Input: part model. Units: mm. Frame: model coordinates. A direction names the side the tool comes from. Coordinates: 2 decimals unless noted, no trailing zeros. Loops run counter-clockwise (first coordinate to the right, second up) from the corner with the lowest first, then second, coordinate; pieces in that order, holes last.
Item 1: Section A-A on x = 32. Return loops of the section in (y, z), and give its area (3 significant figures).
Item 2: Reachability of faces 5 (the cylindrical face through (11.155, 12.58, 2.696)), 6 (the flat face through (38, 8, 3)), 7 (the flat face through (30, 8, 6.35)) from +Z, -Z, +X, -X, +Y, -Y: full face, straight path, thin tool, end or side. Return the list, or none.
Item 3: Section B-B on y = 7.5. Return loops of the section in (x, z).
Item 4: Section D-D on y = 13. Return loops of the section in (x, z) (3 decimals), and give its area (3 significant figures).
Item 5: Ray query, line 1 along Y through (x, z) = (40, 6); line 2 along X through (y, z) = (5.5, 1.5); line 3 along Z through (x, y) = (10, 13.4) (3 decimals). Return the intervals inside material, ascending.
Item 6: Contact query for a flat-ended pin moving along its axis: P1, Ø3, axis at x = 32, y = 2, coming from the +Z side. Output: stop coordinate, or through.
Item 7: Pull-direction query (Y, two-part tool) for faces 1 (the cylindrical face through (51.192, 12.58, 3.55)), 2 (the flat face through (30, 0, 3)), 3 (the flat face through (30, 15, 3)), 4 (the flat face through (39, 3.769, 3)); classes: released by +Y, released by -Y, zero draft, split by the parting line, or undercut.
Item 8: Section C-C on x = 40.5. Return loops of the section in (y, z), and give its area (4 significant figures).
```python
from build123d import *

# Parameters (mm, degrees)
SKETCH1_W             = 60
SKETCH1_H             = 15
SKETCH1_R             = 3
BOSS_EXTRUDE1_DEPTH   = 6.35
M3_TAPPED_HOLE1_D     = 2.5
M3_TAPPED_HOLE1_DEPTH = 8.5
M3_TAPPED_HOLE1_TIP   = 0.751075774
SKETCH5_W             = 3
SKETCH5_H             = 8
CUT_EXTRUDE1_DEPTH    = 63.171717881
M3_TAPPED_HOLE2_D     = 2.5


with BuildPart() as part:
    # Sketch1 → Boss-Extrude1 (new body)
    with BuildSketch(Plane.XY):
        with Locations((30, 7.5)):
            Rectangle(SKETCH1_W, SKETCH1_H)
        with Locations((10, 7.5)):
            Circle(SKETCH1_R, mode=Mode.SUBTRACT)
        with Locations(Location((50, 7.5, 0), (0, 0, 180))):
            Circle(SKETCH1_R, mode=Mode.SUBTRACT)
    extrude(amount=BOSS_EXTRUDE1_DEPTH)

    # M3 Tapped Hole1
    with Locations(Plane(origin=(0, 15, 0), x_dir=(-1, 0, 0), z_dir=(0, 1, 0))):
        with Locations((-10, 3.175), (-50, 3.175)):
            Hole(M3_TAPPED_HOLE1_D / 2, depth=M3_TAPPED_HOLE1_DEPTH)
            with Locations((0, 0, -(M3_TAPPED_HOLE1_DEPTH + M3_TAPPED_HOLE1_TIP / 2))):  # 118° drill point
                Cone(0, M3_TAPPED_HOLE1_D / 2, M3_TAPPED_HOLE1_TIP, mode=Mode.SUBTRACT)

    # Sketch5 → Cut-Extrude1 (cut, through all)
    with BuildSketch(Plane.XY.offset(6.35)):
        with Locations((39.5, 7.769310746)):
            Rectangle(SKETCH5_W, SKETCH5_H)
    extrude(amount=-CUT_EXTRUDE1_DEPTH, mode=Mode.SUBTRACT)

    # M3 Tapped Hole2 (through all)
    with Locations(Plane.XY.offset(6.35)):
        with Locations((32, 13), (32, 2)):
            Hole(M3_TAPPED_HOLE2_D / 2)


solid = part.part
```
Results found:
1. outline: (0, 0) - (0.75, 0) - (0.75, 6.35) - (0, 6.35) - close; (3.25, 0) - (11.75, 0) - (11.75, 6.35) - (3.25, 6.35) - close; (14.25, 0) - (15, 0) - (15, 6.35) - (14.25, 6.35) - close
1. area: 63.5 mm2
2. face 5: +Y
2. face 6: +Z, -Z
2. face 7: +Z, +X, -X, +Y, -Y
3. outline: (0, 0) - (7, 0) - (7, 6.35) - (0, 6.35) - close; (13, 0) - (38, 0) - (38, 6.35) - (13, 6.35) - close; (41, 0) - (47, 0) - (47, 6.35) - (41, 6.35) - close; (53, 0) - (60, 0) - (60, 6.35) - (53, 6.35) - close
4. outline: (0, 0) - (30.75, 0) - (30.75, 6.35) - (0, 6.35) - close; (33.25, 0) - (60, 0) - (60, 6.35) - (33.25, 6.35) - close; hole circle Ø2.5 at (10, 3.175); hole circle Ø2.5 at (50, 3.175)
4. area: 355 mm2
5. line 1: y = 0 to 3.77, 11.77 to 15
5. line 2: x = 0 to 7.76, 12.24 to 38, 41 to 47.76, 52.24 to 60
5. line 3: z = 0 to 1.925, 4.425 to 6.35
6. P1: stops at z = 6.35
7. face 1: zero draft
7. face 2: released by -Y
7. face 3: released by +Y
7. face 4: undercut
8. outline: (0, 0) - (3.77, 0) - (3.77, 6.35) - (0, 6.35) - close; (11.77, 0) - (15, 0) - (15, 6.35) - (11.77, 6.35) - close
8. area: 44.45 mm2
